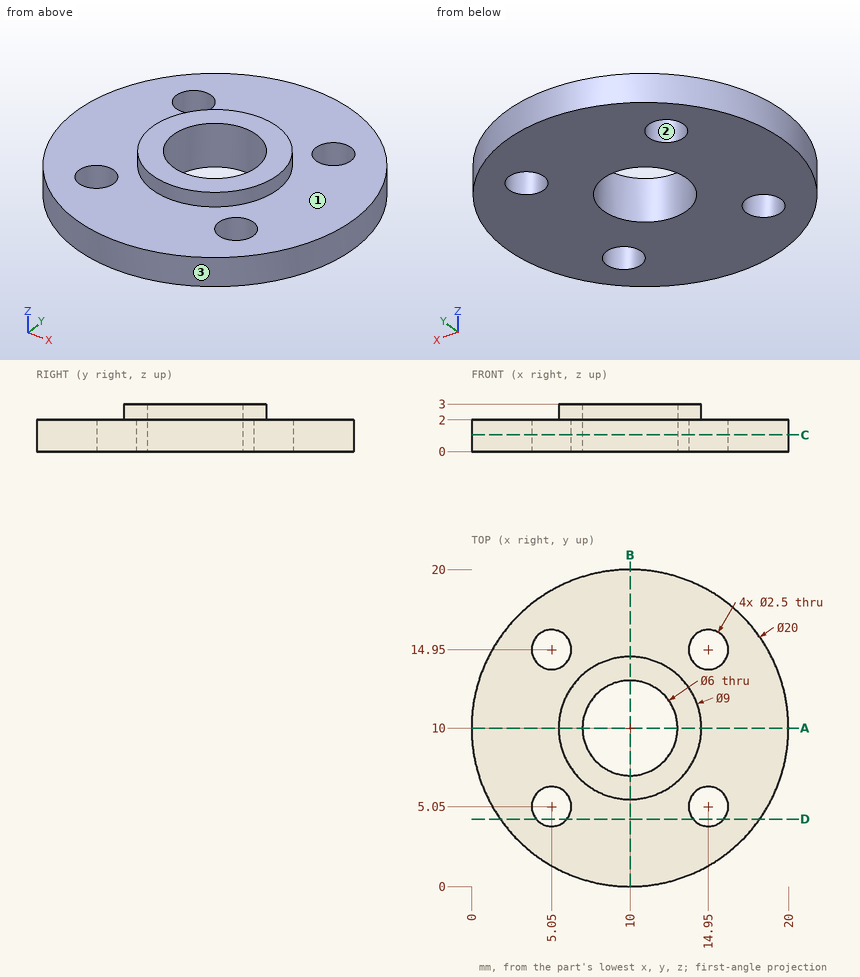
Here's the drawing with two shaded views (mm, measured from the low corner). I have some questions. Give positions to 0.01 mm unless a question says otherwise; leave off trailing zeros. Loops run counter-clockwise (first coordinate to the right, second up) from the corner with the lowest first, then second, coordinate; pieces in that order, holes last. Notation, with made-up numbers: M 85.5,80.5 L 135.5,80.5 A34 ccw 135.5,112.5 Z; hole C -38,0.5 d11. An arc over 180 degrees is marked long. Use one line per item in the form item = value. Start each with the question number.
(1) I want a section at C-C, the plane z = 1.05. Write out the boundary of the cut face in (x, y), and give its area (3 significant figures).
(2) I want a section at D-D, the plane y = 4.25. Write out the boundary of the cut face in (x, z).
(3) I want a section at A-A, the plane y = 10. Write out the boundary of the cut face in (x, z), and give its area (3 significant figures).
(4) Thinking about a two-plate mould opening in Y: for the marked faces 1, 2 and 3, which applies, released by +Y, released by -Y, zero draft, split by the parting line, or undercut?
(5) Please list where these lines run through material, in increasing order: line 1 (Y direction, x = 10, z = 2.2); line 2 (Z direction, x = 6.25, y = 3.75); line 3 (Y direction, x = 14, z = 0.35) (1 decimal).
(6) I'm going to push flat-ended pins straight in: P1, Ø1, axis at x = 12.5, y = 5.5, coming from the -Z side; P2, Ø3, axis at x = 5, y = 2, coming from the +Z side; P3, Ø1, axis at x = 12, z = 2, coming from the -Y side. Where does each tip first touch, or does it pass through?
Worked out:
q1.outline = C 10,10 d20; hole C 5.05,5.05 d2.5; hole C 5.05,14.95 d2.5; hole C 10,10 d6; hole C 14.95,5.05 d2.5; hole C 14.95,14.95 d2.5
q1.area = 266 mm²
q2.outline = M 1.82,0 L 4.09,0 L 4.09,2 L 1.82,2 Z; M 6.01,0 L 13.99,0 L 13.99,2 L 6.01,2 Z; M 15.91,0 L 18.18,0 L 18.18,2 L 15.91,2 Z
q3.outline = M 0,0 L 7,0 L 7,3 L 5.5,3 L 5.5,2 L 0,2 Z; M 13,0 L 20,0 L 20,2 L 14.5,2 L 14.5,3 L 13,3 Z
q3.area = 31.0 mm²
q4.face_1 = zero draft
q4.face_2 = undercut
q4.face_3 = split by the parting line
q5.line_1 = 5.5 to 7, 13 to 14.5
q5.line_2 = 0 to 2
q5.line_3 = 0.8 to 4.2, 5.9 to 14.1, 15.8 to 19.2
q6.P1 = 0
q6.P2 = 2
q6.P3 = 0.11
